Autodesk Inventor part; units mm, degrees
ref_plane "YZ Plane" through (0, 0, 0) normal (1, 0, 0) x (0, 1, 0)
ref_plane "XZ Plane" through (0, 0, 0) normal (0, 1, 0) x (-1, 0, 0)
ref_plane "XY Plane" through (0, 0, 0) normal (0, 0, 1) x (1, 0, 0)
sketch "Sketch1" plane through (0, 0, 0) normal (0, 0, 1) x (1, 0, 0)
  circle A0 centre (0, 0) radius 25
  line L0 (15, -5) -> (35, -5)
  line L1 (35, -5) -> (35, 5)
  line L2 (35, 5) -> (15, 5)
  line L3 (15, 5) -> (15, -5)
  line L4 (15, -5) -> (35, 5) construction
  line L5 (35, -5) -> (15, 5) construction
  point P0 (25, 0)
  dimension "d0" = 50
  dimension "d3" = 10
  dimension "d4" = 20
  dimension "d5" = 0
extrude "Extrusion1" add sketch "Sketch1" along normal mid plane 10 contours A0 L0 L3 L2 | L2 L3 L0 A0
extrude "Extrusion2" add sketch "Sketch1" along normal mid plane 10 contours A0 L0 L3 L2 | A0 L2 L1 L0 picked at (18.3333, 0)
chamfer "Chamfer1" distance 7 angle 20 1 edges at (35, 0, 5) measured on face at (6.5398, 14.4203, 5)
sketch "Sketch2" plane through (28, -5, 5) normal (0.3420201, 0, 0.9396926) x (0.9396926, 0, -0.3420201)
  line L0 (7.4492, 0) -> (0, 0)
  line L1 (0, 0) -> (0, 10)
  line L2 (0, 10) -> (7.4492, 10)
  line L3 (7.4492, 10) -> (7.4492, 0)
  line L4 (7.4492, 0) -> (0, 10) construction
  line L5 (0, 0) -> (7.4492, 10) construction
  line L6 (0, 10) -> (0, 0)
  line L7 (7.4492, 0) -> (7.4492, 10)
  line L8 (7.4492, 10) -> (0, 10)
  line L9 (0, 0) -> (7.4492, 0)
  point P0 (-24.6013, 5)
  point P1 (3.7246, 5)
  dimension "d11" = 0
  dimension "d12" = 0
  dimension "d13" = 0
  dimension "d14" = 0
extrude "Extrusion3" add sketch "Sketch2" along normal blind 10
sketch "Sketch3" plane through (28, -5, 5) normal (-0.9396926, 0, 0.3420201) x (0.3420201, 0, 0.9396926)
  circle A0 centre (5, 5) radius 3.5
  line L0 (10, 10) -> (10, 0)
  line L1 (0, 10) -> (0, 0)
  line L2 (0, 0) -> (10, 0)
  line L3 (0, 10) -> (10, 10)
  point P0 (-14.275, 5)
  dimension "d17" = 7
  dimension "d18" = 5
  dimension "d19" = 5
  dimension "d20" = 5
  dimension "d21" = 5
extrude "Extrusion5" cut sketch "Sketch3" against normal blind 3 contours A0
sketch "Sketch4" plane through (32.5292, 0, 8.6724) normal (-0.9396926, 0, 0.3420201) x (0.3420201, 0, 0.9396926)
  circle A0 centre (0, 0) radius 2.5
  circle A1 centre (0, 0) radius 3.5
  point P0 (-19.275, 0)
  dimension "d32" = 5
extrude "Extrusion6" cut sketch "Sketch4" against normal through all contours A0
chamfer "Chamfer3" distance 5.5 angle 45 1 edges at (35, 0, -5)
sketch "Sketch5" plane through (35, -5, 2.4522) normal (0.9396926, 0, -0.3420201) x (-0.3420201, 0, -0.9396926)
  circle A0 centre (-5, 5) radius 3.5
  circle A1 centre (-5, 5) radius 2.5
  point P0 (14.275, 5)
  dimension "d35" = 7
extrude "Extrusion7" cut sketch "Sketch5" against normal blind 3
pattern_circular "Circular Pattern1" count 3 over 360 about axis through (0, 0, 0) along (0, 0, 1) of "Extrusion3", "Extrusion2", "Chamfer1", "Extrusion5", "Extrusion6", "Extrusion7", "Chamfer3"
equation "\"d18\" = d19"
equation "\"d20\" = d21"
properties part number "BottomPlatform"
Verification items for the finished model (mm, model axes). A direction names the side the tool comes from. Coordinates: 2 decimals unless noted, no trailing zeros. Write each loop counter-clockwise with the first axis right and the second up, starting at its lowest first coordinate (ties: lowest second). Pieces come first, ordered by that corner, then holes. Notation, with made-up numbers: M 6,22 L 40,22 A24 ccw 40,52 Z; hole C 58.5,-4.75 d5. An arc over 180 degrees is marked long. One line per item, written item: value.
Item 1: Section check C-C, the plane z = 9. State how many separate pieces and enclosed holes the cut face has, plus the area to 3 significant figures.
Check sheet entries:
separate pieces: 6
enclosed holes: 0
area: 87.8 mm^2
Item 2: Section check B-B, the plane x = 15. Record the boundary of the cut face in (y, z), plus the area to 3 significant figures.
Check sheet entries:
outline: M -20,-5 L 20,-5 L 20,5 L -20,5 Z
area: 400 mm^2
Item 3: Mould release check, pull along Y, two halves, no side actions. Record for faces 1 (the flat face through (33.312, -1.507, 10.818)), 2 (the flat face through (-16.2, -27.93, -2.21)), 3 (the flat face through (-17.439, 30.346, 1.462)): pulls with the +Y half, pulls with the -Y half, needs draft (parallel to the pull), parting line crosses it, or undercut.
Check sheet entries:
face 1: undercut
face 2: pulls with the -Y half
face 3: pulls with the +Y half
Item 4: Scan lines: line 1 along Y through (x, z) = (35.5, 12); line 2 along X through (y, z) = (-31, 9.5). Record each from-to range of solid material in increasing order.
Check sheet entries:
line 1: y = -5 to 5
line 2: x = -21.44 to -20.84, -15.05 to -12.12
Item 5: Gauge pin test, flat ends, axial feed: pin 1 Ø8 at (x, y) = (-12.5, 5.5) entering from +Z; pin 2 Ø2 at (x, z) = (8, 4.5) entering from +Y; pin 3 Ø6 at (y, z) = (6, 7) entering from -X. Record the tip position at first contact, or that the pin passes through.
Check sheet entries:
pin 1: stops at z = 5
pin 2: stops at y = 24
pin 3: stops at x = -24.72
Item 6: Section check D-D, the plane y = 10.5. Record the boundary of the cut face in (x, z).
Check sheet entries:
outline: M -22.69,-5 L 22.69,-5 L 22.69,5 L -22.69,5 Z
Item 7: Access from +Z, -Z, +X, -X, +Y, -Y to the whole of each face (thin tool, end or side, straight path). Record for faces 4 (the flat face through (-19.4, -23.6, 3.7)), 5 (the flat face through (-14.709, 30.045, 6.762)), 6 (the flat face through (28.546, -2.292, 6.5)), 7 (the flat face through (32.3, -0.1, -2.2)).
Check sheet entries:
face 4: +Z, -Z, -X
face 5: none
face 6: +Z, -X, +Y, -Y
face 7: -Z, +X, +Y, -Y
Item 8: Section check A-A, the plane z = -0.75. Record the boundary of the cut face in (x, y).
Check sheet entries:
outline: M -21.21,-26.73 L -12.54,-31.73 L -7.92,-23.71 A25 ccw 24.49,-5 L 33.75,-5 L 33.75,5 L 24.49,5 A25 ccw -7.92,23.71 L -12.54,31.73 L -21.21,26.73 L -16.58,18.71 A25 ccw -16.58,-18.71 Z
